```python
from build123d import *

# Parameters (mm, degrees)
F0_R     = 215.9
F1_DEPTH = 336.55
F2_T     = -6.35
F3_R     = 19.05
F4_DEPTH = 254


with BuildPart() as f1:
    # F0 (on Top) → F1 (new body)
    with BuildSketch(Plane.XY):
        Circle(F0_R)
    extrude(amount=F1_DEPTH)

    # F2
    f2_openings = [f1.faces().sort_by_distance(p)[0] for p in [
        (0, 0, 336.55),
        (0, 0, 0),
    ]]
    offset(amount=F2_T, openings=f2_openings)

    # F3 (on Front) → F4 (cut, symmetric)
    with BuildSketch(Plane.XZ):
        with Locations((0, 241.3)):
            Circle(F3_R)
    extrude(amount=F4_DEPTH, both=True, mode=Mode.SUBTRACT)


solid = f1.part
```
Geometry: final body of the model. Coordinates: model frame, mm. Coordinates: 2 decimals unless noted, no trailing zeros. Loops run counter-clockwise (first coordinate to the right, second up) from the corner with the lowest first, then second, coordinate; pieces in that order, holes last. Notation, with made-up numbers: (-28.75, 7.5) -> (-7.75, 7.5) arc R25 cw to (-7.75, 28.5) -> close; hole circle Ø11 at (59, -32). An arc over 180 degrees is marked (long way). Use a Markdown table: item, result. Add a question column.
(1) Line query: line 1 along Z through (x, y) = (0, 211); line 2 along X through (y, z) = (166.5, 244); line 3 along Y through (x, z) = (188.5, 188). Output: solid intervals per line, ascending.
(2) Mould query, pull axis X, two halves, no side actions, for faces 1 (the cylindrical face through (-159.127, 145.915, 165.919)), 2 (the flat face through (-113, 177, 0)), 3 (the cylindrical face through (8.79, -212.34, 224.4)), 4 (the cylindrical face through (8.79, 212.24, 224.4)). Classes: pulls with the +X half, pulls with the -X half, needs draft (parallel to the pull), parting line crosses it, or undercut.
(3) Pin query (flat end, axial travel): pin 1 Ø8 at (x, z) = (46, 84.5) entering from +Y; pin 2 Ø12 at (x, z) = (-170.5, 198.5) entering from +Y; pin 3 Ø5 at (y, z) = (-70.5, 76.5) entering from +X. Return the tip coordinate at first contact, or that it passes through.
(4) Section query B-B, the plane y = 0. Return loops of the section in (x, z).
(5) Section query A-A, the plane x = 0. Return loops of the section in (y, z).
(6) Section query D-D, the plane z = 137.5. Return loops of the section in (x, y), plus the area to 3 significant figures.
(7) Section query C-C, the plane z = 241.3. Return loops of the section in (x, y).
Answer:
| question | item | result |
|---|---|---|
| 1 | line 1 | z = 0 to 222.25, 260.35 to 336.55 |
| 1 | line 2 | x = -137.44 to -127.24, 127.24 to 137.44 |
| 1 | line 3 | y = -105.26 to -91.54, 91.54 to 105.26 |
| 2 | face 1 | parting line crosses it |
| 2 | face 2 | needs draft |
| 2 | face 3 | undercut |
| 2 | face 4 | undercut |
| 3 | pin 1 | stops at y = 211.78 |
| 3 | pin 2 | stops at y = 139.83 |
| 3 | pin 3 | stops at x = 204.91 |
| 4 | outline | (-215.9, 0) -> (-209.55, 0) -> (-209.55, 336.55) -> (-215.9, 336.55) -> close; (209.55, 0) -> (215.9, 0) -> (215.9, 336.55) -> (209.55, 336.55) -> close |
| 5 | outline | (-215.9, 0) -> (-209.55, 0) -> (-209.55, 222.25) -> (-215.9, 222.25) -> close; (-215.9, 260.35) -> (-209.55, 260.35) -> (-209.55, 336.55) -> (-215.9, 336.55) -> close; (209.55, 0) -> (215.9, 0) -> (215.9, 222.25) -> (209.55, 222.25) -> close; (209.55, 260.35) -> (215.9, 260.35) -> (215.9, 336.55) -> (209.55, 336.55) -> close |
| 6 | outline | circle Ø431.8 at (0, 0); hole circle Ø419.1 at (0, 0) |
| 6 | area | 8,490 mm^2 |
| 7 | outline | (-19.05, -215.06) -> (-19.05, -208.68) arc R209.55 cw to (-19.05, 208.68) -> (-19.05, 215.06) arc R215.9 ccw to start; (19.05, -215.06) arc R215.9 ccw to (19.05, 215.06) -> (19.05, 208.68) arc R209.55 cw to (19.05, -208.68) -> close |
